Geometry: final body of the model. Coordinates: model frame, mm. Face numbers are marked on the shaded views. A direction names the side the tool comes from. Give positions to 0.01 mm unless a question says otherwise; leave off trailing zeros.
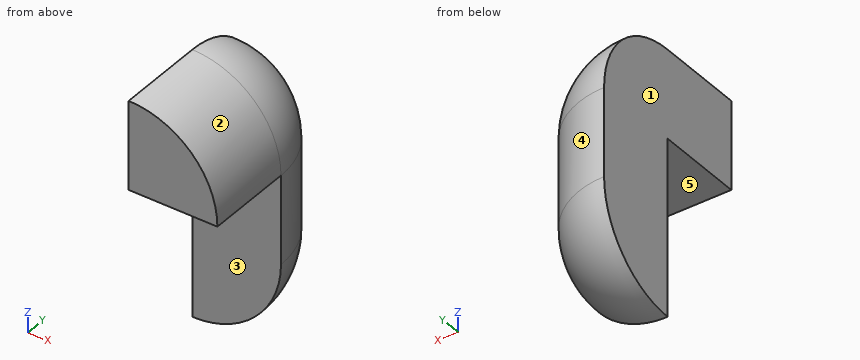
```python
from build123d import *

# Parameters (mm, degrees)
F0_W     = 25.4
F0_H     = 25.4
F1_DEPTH = 76.2
F2_W     = 25.4
F2_H     = 25.4
F3_DEPTH = 25.4
F4_R     = 25.39999


# Not quite as in the source:
# - a fillet or chamfer is up to 0.001 mm smaller than in the source, because OpenCascade refuses the exact size


with BuildPart() as f1:
    # F0 (on Top) → F1 (new body)
    with BuildSketch(Plane.XY):
        with Locations((12.7, 12.7)):
            Rectangle(F0_W, F0_H)
    extrude(amount=F1_DEPTH)

    # F2 (on face) → F3 (join)
    with BuildSketch(Plane.XZ):
        with Locations((12.7, 63.5)):
            Rectangle(F2_W, F2_H)
    extrude(amount=F3_DEPTH)

    # F4 (radius 25.4 in the source; OpenCascade refuses exactly that, so slightly less here)
    f4_edges = [f1.edges().sort_by_distance(p)[0] for p in [
        (12.7, 25.4, 0),
        (25.4, 12.7, 0),
        (25.4, 25.4, 38.1),
        (25.4, 0, 76.2),
        (12.7, 25.4, 76.2),
    ]]
    fillet(f4_edges, radius=F4_R)


solid = f1.part
```
Item 1: Reachability of the marked faces 4 and 5 from +Z, -Z, +X, -X, +Y, -Y: full face, straight path, thin tool, end or side. Return the list, or none.
Found:
face 4: +Z, -Z, +X, +Y
face 5: -Z, +X, -X, -Y
Item 2: Pull-direction query (X, two-part tool) for the marked faces 1, 2 and 3; classes: +X half, -X half, draft (parallel to the pull), parting line (faces both ways), or undercut.
Found:
face 1: -X half
face 2: +X half
face 3: draft
Item 3: Line query: L1, parallel to Y at x = 6, z = 57; L2, parallel to Z at x = 5.75, y = -21; L3, parallel to Z at x = 19.25, y = 9.5. Output: solid intervals per line, ascending.
Found:
L1: y = -25.4 to 23.89
L2: z = 50.8 to 75.54
L3: z = 11.82 to 64.38
Item 4: Pin query (flat end, axial travel): pin 1 Ø1.5 at (y, z) = (-3.5, 51.5) entering from +X; pin 2 Ø12 at (x, z) = (15, 20.5) entering from -Y; pin 3 Ø7.5 at (x, y) = (7, -8) entering from -Z; pin 4 Ø1.5 at (x, z) = (17, 18) entering from +Y. Return the tip coordinate at first contact, or that it passes through.
Found:
pin 1: stops at x = 25.4
pin 2: stops at y = 0
pin 3: stops at z = 50.8
pin 4: stops at y = 18.13
